```python
from build123d import *

# Parameters (mm, degrees)
SKETCH1_W           = 198.979955438
SKETCH1_H           = 42.541825
SKETCH1_R           = 2.2479
BOSS_EXTRUDE1_DEPTH = 9.525
SKETCH1_5_R         = 2.2479
CUT_EXTRUDE1_DEPTH  = 6.35
CUT_EXTRUDE2_DEPTH  = 196.596168108


with BuildPart() as part:
    # Sketch1 → Boss-Extrude1 (new body)
    with BuildSketch(Plane(origin=(0, 0, 0), x_dir=(1, 0, 0), z_dir=(0, 1, 0))):
        with Locations((91.186, 21.2709125)):
            Rectangle(SKETCH1_W, SKETCH1_H)
        with Locations(Location((45.72, 38.1, 0), (0, 0, 270))):
            Circle(SKETCH1_R, mode=Mode.SUBTRACT)
        with Locations(Location((38.1, 38.1, 0), (0, 0, 270))):
            Circle(SKETCH1_R, mode=Mode.SUBTRACT)
        with Locations(Location((30.48, 38.1, 0), (0, 0, 270))):
            Circle(SKETCH1_R, mode=Mode.SUBTRACT)
        with Locations(Location((22.86, 38.1, 0), (0, 0, 270))):
            Circle(SKETCH1_R, mode=Mode.SUBTRACT)
        with Locations(Location((15.24, 38.1, 0), (0, 0, 270))):
            Circle(SKETCH1_R, mode=Mode.SUBTRACT)
        with Locations(Location((7.62, 38.1, 0), (0, 0, 270))):
            Circle(SKETCH1_R, mode=Mode.SUBTRACT)
        with Locations(Location((0, 38.1, 0), (0, 0, 270))):
            Circle(SKETCH1_R, mode=Mode.SUBTRACT)
        with Locations(Location((53.34, 38.1, 0), (0, 0, 270))):
            Circle(SKETCH1_R, mode=Mode.SUBTRACT)
        with Locations(Location((157.988, 38.1, 0), (0, 0, 270))):
            Circle(SKETCH1_R, mode=Mode.SUBTRACT)
        with Locations(Location((149.86, 38.1, 0), (0, 0, 270))):
            Circle(SKETCH1_R, mode=Mode.SUBTRACT)
        with Locations(Location((141.732, 38.1, 0), (0, 0, 270))):
            Circle(SKETCH1_R, mode=Mode.SUBTRACT)
        with Locations(Location((133.604, 38.1, 0), (0, 0, 270))):
            Circle(SKETCH1_R, mode=Mode.SUBTRACT)
        with Locations(Location((125.476, 38.1, 0), (0, 0, 270))):
            Circle(SKETCH1_R, mode=Mode.SUBTRACT)
        with Locations(Location((166.116, 38.1, 0), (0, 0, 270))):
            Circle(SKETCH1_R, mode=Mode.SUBTRACT)
        with Locations(Location((174.244, 38.1, 0), (0, 0, 270))):
            Circle(SKETCH1_R, mode=Mode.SUBTRACT)
        with Locations(Location((182.372, 38.1, 0), (0, 0, 270))):
            Circle(SKETCH1_R, mode=Mode.SUBTRACT)
    extrude(amount=-BOSS_EXTRUDE1_DEPTH)

    # Sketch1<5> → Cut-Extrude1 (cut)
    # profile 1 of 2: a face of its own
    with BuildSketch(Plane(origin=(0, 0, 0), x_dir=(1, 0, 0), z_dir=(0, 1, 0))):
        Polygon((-5.128977719, 38.1), (-2.564488859, 33.658175), (2.564488859, 33.658175), (3.81, 35.815463577), (5.055511141, 33.658175), (10.184488859, 33.658175), (11.43, 35.815463577), (12.675511141, 33.658175), (17.804488859, 33.658175), (19.05, 35.815463577), (20.295511141, 33.658175), (25.424488859, 33.658175), (26.67, 35.815463577), (27.915511141, 33.658175), (33.044488859, 33.658175), (34.29, 35.815463577), (35.535511141, 33.658175), (40.664488859, 33.658175), (41.91, 35.815463577), (43.155511141, 33.658175), (48.284488859, 33.658175), (49.53, 35.815463577), (50.775511141, 33.658175), (55.904488859, 33.658175), (58.468977719, 38.1), (58.468977719, 42.541825), (-5.128977719, 42.541825), align=None)
        with Locations((0, 38.1)):
            Circle(SKETCH1_5_R, mode=Mode.SUBTRACT)
        with Locations((7.62, 38.1)):
            Circle(SKETCH1_5_R, mode=Mode.SUBTRACT)
        with Locations((15.24, 38.1)):
            Circle(SKETCH1_5_R, mode=Mode.SUBTRACT)
        with Locations((22.86, 38.1)):
            Circle(SKETCH1_5_R, mode=Mode.SUBTRACT)
        with Locations((30.48, 38.1)):
            Circle(SKETCH1_5_R, mode=Mode.SUBTRACT)
        with Locations((38.1, 38.1)):
            Circle(SKETCH1_5_R, mode=Mode.SUBTRACT)
        with Locations((45.72, 38.1)):
            Circle(SKETCH1_5_R, mode=Mode.SUBTRACT)
        with Locations((53.34, 38.1)):
            Circle(SKETCH1_5_R, mode=Mode.SUBTRACT)
    # profile 2 of 2: a face of its own
    with BuildSketch(Plane(origin=(0, 0, 0), x_dir=(1, 0, 0), z_dir=(0, 1, 0))):
        Polygon((179.807511141, 33.658175), (184.936488859, 33.658175), (187.500977719, 38.1), (187.500977719, 42.541825), (120.347022281, 42.541825), (120.347022281, 38.1), (122.911511141, 33.658175), (128.040488859, 33.658175), (129.54, 36.255404482), (131.039511141, 33.658175), (136.168488859, 33.658175), (137.668, 36.255404482), (139.167511141, 33.658175), (144.296488859, 33.658175), (145.796, 36.255404482), (147.295511141, 33.658175), (152.424488859, 33.658175), (153.924, 36.255404482), (155.423511141, 33.658175), (160.552488859, 33.658175), (162.052, 36.255404482), (163.551511141, 33.658175), (168.680488859, 33.658175), (170.18, 36.255404482), (171.679511141, 33.658175), (176.808488859, 33.658175), (178.308, 36.255404482), align=None)
        with Locations((125.476, 38.1)):
            Circle(SKETCH1_5_R, mode=Mode.SUBTRACT)
        with Locations((133.604, 38.1)):
            Circle(SKETCH1_5_R, mode=Mode.SUBTRACT)
        with Locations((141.732, 38.1)):
            Circle(SKETCH1_5_R, mode=Mode.SUBTRACT)
        with Locations((149.86, 38.1)):
            Circle(SKETCH1_5_R, mode=Mode.SUBTRACT)
        with Locations((157.988, 38.1)):
            Circle(SKETCH1_5_R, mode=Mode.SUBTRACT)
        with Locations((166.116, 38.1)):
            Circle(SKETCH1_5_R, mode=Mode.SUBTRACT)
        with Locations((174.244, 38.1)):
            Circle(SKETCH1_5_R, mode=Mode.SUBTRACT)
        with Locations((182.372, 38.1)):
            Circle(SKETCH1_5_R, mode=Mode.SUBTRACT)
    extrude(amount=-CUT_EXTRUDE1_DEPTH, mode=Mode.SUBTRACT)

    # Mirror1: part across plane


with BuildPart() as part_1:
    add(part.part)
    add(part.part.mirror(Plane.XY))

    # Sketch2 → Cut-Extrude2 (cut, through all)
    with BuildSketch(Plane(origin=(0, 0, 0), x_dir=(1, 0, 0), z_dir=(0, 1, 0))):
        with BuildLine():
            Line((157.988, -19), (149.86, -19))
            ThreePointArc((149.86, -19), (130.86, 0), (149.86, 19))
            Line((149.86, 19), (157.988, 19))
            ThreePointArc((157.988, 19), (176.988, 0), (157.988, -19))
        make_face()
        with BuildLine():
            Line((28.956, -19), (24.384, -19))
            ThreePointArc((24.384, -19), (5.384, 0), (24.384, 19))
            Line((24.384, 19), (28.956, 19))
            ThreePointArc((28.956, 19), (47.956, 0), (28.956, -19))
        make_face()
    extrude(amount=-CUT_EXTRUDE2_DEPTH, mode=Mode.SUBTRACT)


solid = part_1.part
```
Could you check a few things on this model? Use its own coordinates, in mm. A direction names the side the tool comes from. Coordinates: 2 decimals unless noted, no trailing zeros. Order: outer loops, then holes, each group sorted by start corner. A loop starts at its lowest first (then second) coordinate and runs counter-clockwise, first axis right, second up. Notation, with made-up numbers: M 60,19 L 118,19 A25 cw 118,43 Z; hole C 3.5,14.5 d6. An arc over 180 degrees is marked long. Use a Markdown table: item, result. Add a question column.
Q1. I want a section at C-C on y = -2.5. Give the number of separate pieces and of enclosed holes in the cut face, then the cut area to 3 significant figures.
Q2. Which directions (+Z, -Z, +X, -X, +Y, -Y) give clear straight access to the entire face, cutting with the end or side of a thin tool? Please do faces 5 (the flat face through (190.676, -5, -1)), 6 (the flat face through (187.501, -3, 40)), 7 (the flat face through (27, -5, -19)), 8 (the flat face through (120.347, -3, -40)).
Q3. I want a section at B-B on x = 15.24. List the corners of the cut face in (y, z) for me (3 decimals).
Q4. I want a section at A-A on z = 0. List the corners of the cut face in (x, y) for me (3 decimals).
Q5. I'm going to push flat-ended pins straight in: pin 1 (3.5 mm diameter, centred on x = 53.34, z = 38.1, fed in from +Y); pin 2 (5.5 mm diameter, centred on x = 141.5, y = -4.5, fed in from +Z); pin 3 (2.5 mm diameter, centred on x = 45, y = -2.5, fed in from -Z); pin 4 (5.5 mm diameter, centred on x = 174.5, y = -3.5, fed in from +Z). Where does each tip first touch, or does it pass through?
Q6. We'd pull the mould along Z, two halves only. Please class faces 1 (the flat face through (186.2, -3.13, 35.85)), 2 (the cylindrical face through (174.919, -7.915, -35.956)), 3 (the cylindrical face through (139.74, -7.92, 37.06)), 4 (the flat face through (125, -3, -33.658)): pulls with the +Z half, pulls with the -Z half, needs draft (parallel to the pull), parting line crosses it, or undercut.
Q7. If I drill on L1, parallel to Z at x = 0, y = -8.5; L2, parallel to Z at x = 45.5, y = -6.5; L3, parallel to Z at x = 38.1, y = -8.05, over which ranges is the centre line in solid material (lowest first)?
Checked values:
| question | item | result |
|---|---|---|
| 1 | separate pieces | 1 |
| 1 | enclosed holes | 2 |
| 1 | area | 12,000 mm² |
| 2 | face 5 | +Z, -Z, +X, +Y, -Y |
| 2 | face 6 | +Z, +Y |
| 2 | face 7 | +Y, -Y |
| 2 | face 8 | -Z, +Y |
| 3 | outline | M -9.525,-42.542 L -6.35,-42.542 L -6.35,-40.348 L -9.525,-40.348 Z; M -9.525,-35.852 L -6.35,-35.852 L -6.35,-33.658 L 0,-33.658 L 0,-16.655 L -9.525,-16.655 Z; M -9.525,16.655 L 0,16.655 L 0,33.658 L -6.35,33.658 L -6.35,35.852 L -9.525,35.852 Z; M -9.525,40.348 L -6.35,40.348 L -6.35,42.542 L -9.525,42.542 Z |
| 4 | outline | M -8.304,-9.525 L 5.384,-9.525 L 5.384,0 L -8.304,0 Z; M 47.956,-9.525 L 130.86,-9.525 L 130.86,0 L 47.956,0 Z; M 176.988,-9.525 L 190.676,-9.525 L 190.676,0 L 176.988,0 Z |
| 5 | pin 1 | through |
| 5 | pin 2 | z = 42.54 |
| 5 | pin 3 | z = -33.66 |
| 5 | pin 4 | z = 34.42 |
| 6 | face 1 | pulls with the +Z half |
| 6 | face 2 | undercut |
| 6 | face 3 | undercut |
| 6 | face 4 | pulls with the -Z half |
| 7 | L1 | -42.54 to -40.35, -35.85 to 35.85, 40.35 to 42.54 |
| 7 | L2 | -42.54 to -40.34, -35.86 to -9.34, 9.34 to 35.86, 40.34 to 42.54 |
| 7 | L3 | -42.54 to -40.35, -35.85 to -16.65, 16.65 to 35.85, 40.35 to 42.54 |
